Geometry: final body of the model. Coordinates: model frame, mm. Face numbers are marked on the shaded views. Round coordinates to 2 decimals unless told otherwise and drop trailing zeros. Loops run counter-clockwise (first coordinate to the right, second up) from the corner with the lowest first, then second, coordinate; pieces in that order, holes last. Notation, with made-up numbers: (76, -6) - (121, -6) arc R28 ccw to (121, 19) - close; hole circle Ø9 at (20.5, -34.75). An arc over 180 degrees is marked (long way). Use CSV: the item, a comma, the result in double quotes.
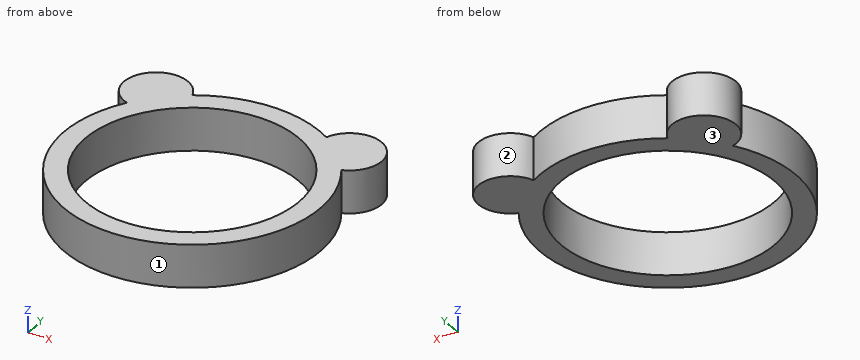
from build123d import *

# Parameters (mm, degrees)
SKETCH_R     = 12
SKETCH_R_2   = 10
PAD_DEPTH    = 4
SKETCH001_R  = 3
PAD001_DEPTH = 4


with BuildPart() as part:
    # Sketch → Pad (new body)
    with BuildSketch(Plane.XY):
        Circle(SKETCH_R)
        Circle(SKETCH_R_2, mode=Mode.SUBTRACT)
    extrude(amount=PAD_DEPTH)

    # Sketch001 → Pad001 (join)
    with BuildSketch(Plane.XY):
        with Locations((-9.192388, 9.192388)):
            Circle(SKETCH001_R)
    pad001 = extrude(amount=PAD001_DEPTH)

    # Mirrored: Pad001 across YZ
    add(pad001.mirror(Plane.YZ))


solid = part.part
Item 1: Section A-A on x = 0. Return the cut outline in (y, z).
Final values:
outline,"(-12, 0) - (-10, 0) - (-10, 4) - (-12, 4) - close; (10, 0) - (12, 0) - (12, 4) - (10, 4) - close"
Item 2: Mould query, pull axis X, two halves, no side actions, for the marked faces 1, 2 and 3. Classes: released by +X, released by -X, zero draft, split by the parting line, or undercut.
Final values:
face 1,"split by the parting line"
face 2,"undercut"
face 3,"zero draft"
Item 3: Material intervals for line 1 (Y direction, x = 3.5, z = 0.5); line 2 (X direction, y = 5, z = 2); line 3 (Y direction, x = 0.75, z = 1.35), sorted ascending.
Final values:
line 1,"y = -11.48 to -9.37, 9.37 to 11.48"
line 2,"x = -10.91 to -8.66, 8.66 to 10.91"
line 3,"y = -11.98 to -9.97, 9.97 to 11.98"
Item 4: Section C-C on z = 0.75. Return the cut outline in (x, y), plus the area to 3 significant figures.
Final values:
outline,"(-10.18, 6.36) arc R12 ccw (long way) to (10.18, 6.36) arc R3 ccw (long way) to (6.36, 10.18) arc R12 ccw to (-6.36, 10.18) arc R3 ccw (long way) to start; hole circle Ø20 at (0, 0)"
area,"179 mm²"
Item 5: Pin query (flat end, axial travel): P1, Ø3, axis at x = 6, y = -7, coming from the +Z side; P2, Ø1.5, axis at y = 6.5, z = 3, coming from the +X side. Return the tip coordinate at first contact, or that it passes through.
Final values:
P1,"stops at z = 4"
P2,"stops at x = 11.48"
